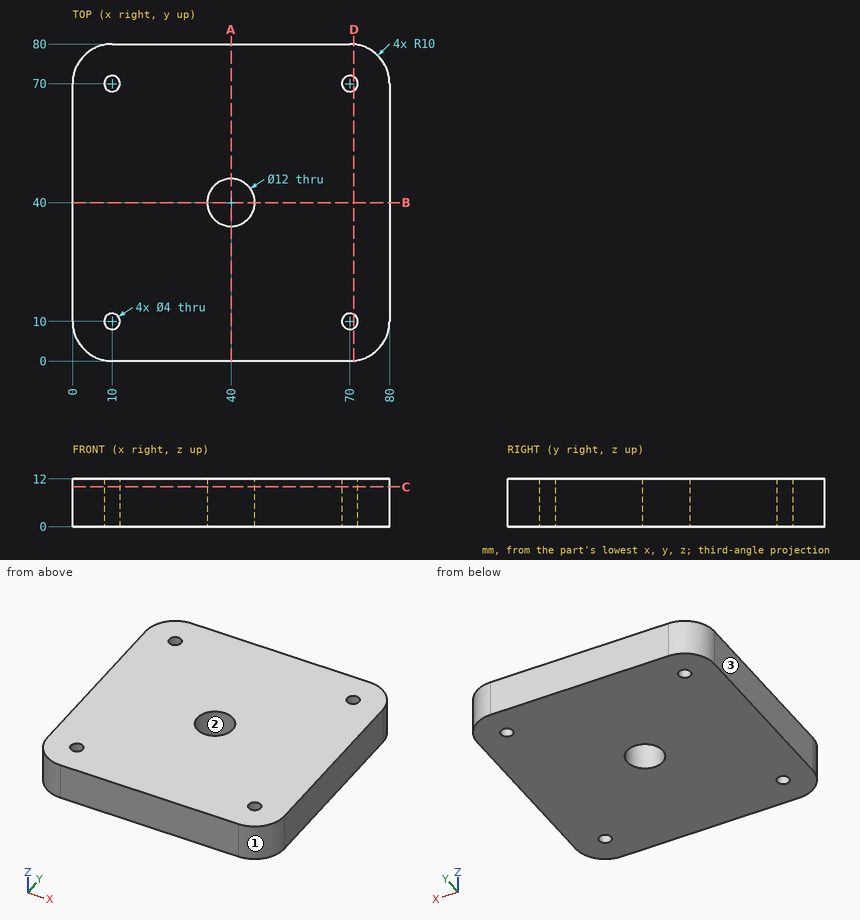
Source: three-view drawing plus pictorial views. Frame: mm from the lowest corner of the part. Round coordinates to 2 decimals unless told otherwise and drop trailing zeros. Loops run counter-clockwise (first coordinate to the right, second up) from the corner with the lowest first, then second, coordinate; pieces in that order, holes last. Notation, with made-up numbers: (-3.5, 55.5) - (1.5, 55.5) arc R15 cw to (1.5, 59.5) - close; hole circle Ø6 at (-36.75, -17). An arc over 180 degrees is marked (long way). Write item = value, one per line. Start each with the question number.
Item 1: Section query D-D on x = 71. Output: boundary loops of the cut face in (y, z), plus the area to 3 significant figures.
Item 2: Section query C-C on z = 10. Output: boundary loops of the cut face in (x, y), plus the area to 3 significant figures.
Item 3: Material intervals for line 1 (Y direction, x = 70, z = 5.75); line 2 (Y direction, x = 40, z = 4); line 3 (X direction, y = 9, z = 3.5), sorted ascending.
Item 4: First-contact query: pin 1 Ø2 at (y, z) = (42.5, 10) entering from -X; pin 2 Ø3 at (x, y) = (70, 10) entering from -Z. Flat tips, straight axial feed; report the tip coordinate or a pass-through.
Item 5: Mould query, pull axis Y, two halves, no side actions, for the marked faces 1, 2 and 3. Classes: released by +Y, released by -Y, zero draft, split by the parting line, or undercut.
Item 6: Section query A-A on x = 40. Output: boundary loops of the cut face in (y, z), plus the area to 3 significant figures.
Results list:
q1.outline = (0.05, 0) - (8.27, 0) - (8.27, 12) - (0.05, 12) - close; (11.73, 0) - (68.27, 0) - (68.27, 12) - (11.73, 12) - close; (71.73, 0) - (79.95, 0) - (79.95, 12) - (71.73, 12) - close
q1.area = 876 mm²
q2.outline = (0, 10) arc R10 ccw to (10, 0) - (70, 0) arc R10 ccw to (80, 10) - (80, 70) arc R10 ccw to (70, 80) - (10, 80) arc R10 ccw to (0, 70) - close; hole circle Ø4 at (10, 10); hole circle Ø4 at (10, 70); hole circle Ø12 at (40, 40); hole circle Ø4 at (70, 10); hole circle Ø4 at (70, 70)
q2.area = 6,150 mm²
q3.line_1 = 0 to 8, 12 to 68, 72 to 80
q3.line_2 = 0 to 34, 46 to 80
q3.line_3 = 0.05 to 8.27, 11.73 to 68.27, 71.73 to 79.95
q4.pin_1 = 0
q4.pin_2 = through
q5.face_1 = released by -Y
q5.face_2 = undercut
q5.face_3 = zero draft
q6.outline = (0, 0) - (34, 0) - (34, 12) - (0, 12) - close; (46, 0) - (80, 0) - (80, 12) - (46, 12) - close
q6.area = 816 mm²
